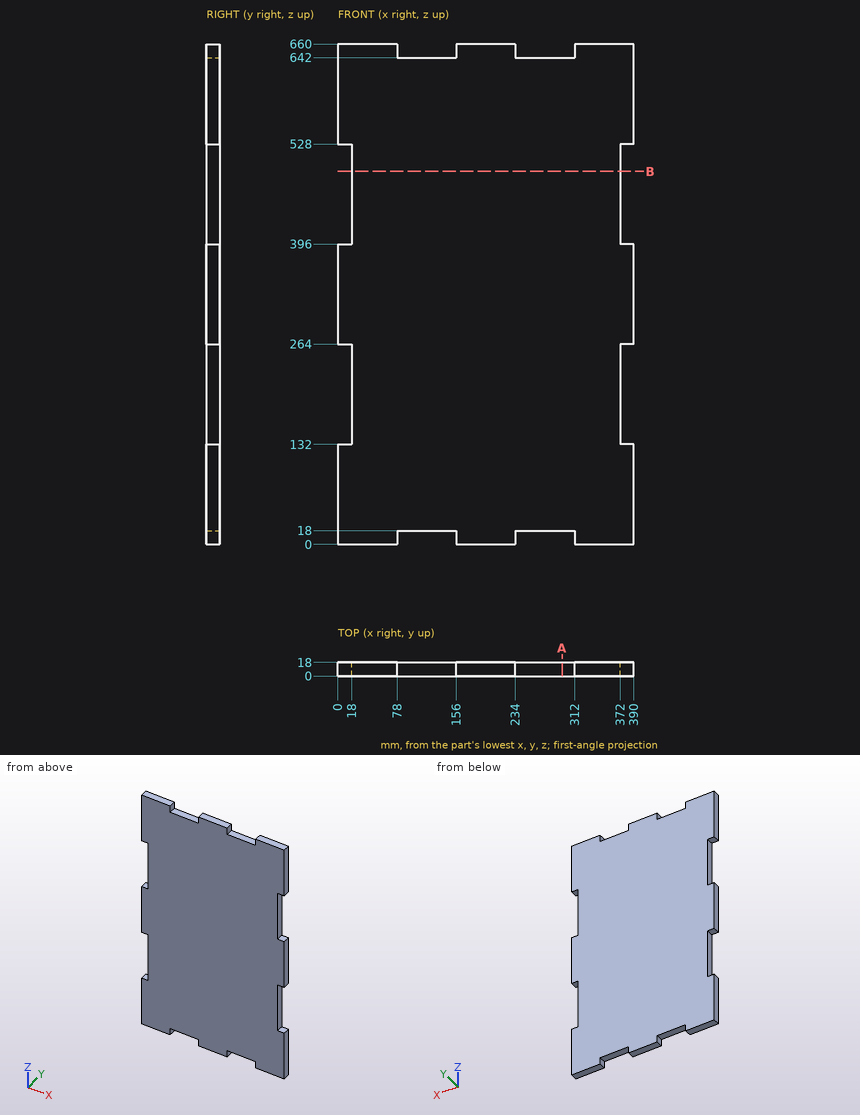
Check sheet for the drawn part. Datum: minimum x, y, z corner. Units: mm. Coordinates: 2 decimals unless noted, no trailing zeros. Order: outer loops, then holes, each group sorted by start corner. A loop starts at its lowest first (then second) coordinate and runs counter-clockwise, first axis right, second up. Notation, with made-up numbers: (-29, 42) - (1, 42) arc R31 ccw to (1, 68) - close; hole circle Ø6 at (25, -32). An arc over 180 degrees is marked (long way). Return JSON: item names as keys, results as strings.
(1) Thickness scan on line 1 along Z through (x, y) = (274.5, 8.75); line 2 along X through (y, z) = (4, 167). Record the ranges inside material, lowest first.
Filled sheet:
{"line 1": "z = 18 to 642", "line 2": "x = 18 to 372"}
(2) Section check B-B, the plane z = 492. Record the cut outline in (x, y).
Filled sheet:
{"outline": "(18, 0) - (372, 0) - (372, 18) - (18, 18) - close"}
(3) Go/stop test with flat-tipped pins: pin 1 (5 mm diameter, centred on x = 291.5, z = 568, fed in from -Y); pin 2 (9 mm diameter, centred on x = 266.5, y = 11, fed in from +Z); pin 3 (9 mm diameter, centred on x = 259, y = 11.5, fed in from -Z); pin 4 (8 mm diameter, centred on y = 2.5, z = 170.5, fed in from -X). Record where each tip stops, or that it passes through.
Filled sheet:
{"pin 1": "stops at y = 0", "pin 2": "stops at z = 642", "pin 3": "stops at z = 18", "pin 4": "stops at x = 18"}
(4) Section check A-A, the plane x = 295.5. Record the cut outline in (y, z), and give its area (3 significant figures).
Filled sheet:
{"outline": "(0, 18) - (18, 18) - (18, 642) - (0, 642) - close", "area": "11,200 mm^2"}
